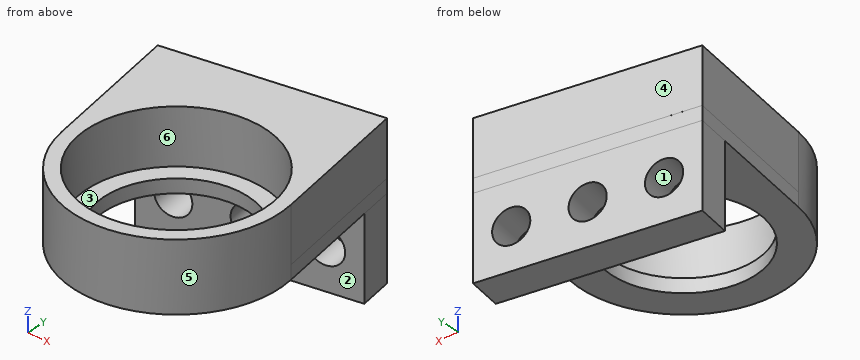
Autodesk Inventor part; units mm, degrees
ref_plane "Work Plane1" through (-17.5555, -24.5446, -8) normal (0, 0, -1) x (0, 1, 0)
ref_plane "YZ Plane" through (0, 0, 0) normal (1, 0, 0) x (0, 1, 0)
ref_plane "XZ Plane" through (0, 0, 0) normal (0, 1, 0) x (-1, 0, 0)
sketch "Sketch1" plane through (0, 0, 0) normal (0, 0, 1) x (1, 0, 0)
  circle A0 centre (0, -6.9891) radius 13
  line L0 (-8.3396, 25.9015) -> (-6.0783, 13.4045)
  line L1 (9.8647, 29.1956) -> (12.126, 16.6985)
  line L2 (-201.5028, -9.0509) -> (9.8647, 29.1956)
  line L3 (-199.2415, -21.5479) -> (-201.5028, -9.0509)
  line L4 (-199.2415, -21.5479) -> (12.126, 16.6985)
  line L5 (0, -6.9891) -> (-3.7659, 13.8229) construction
  circle A1 centre (0, -6.9891) radius 15
  line L6 (0, -6.9891) -> (-14.7603, -9.66) construction
  line L7 (-14.7603, -9.66) -> (-18.5262, 11.1521)
  line L8 (0, -6.9891) -> (14.7603, -4.3183) construction
  line L9 (14.7603, -4.3183) -> (10.9944, 16.4937)
  line L10 (10.9944, 16.4937) -> (-18.5262, 11.1521)
  point P0 (0, 0)
ref_plane "Work Plane1" through (-17.5555, -24.5446, -8) normal (0, 0, -1) x (0, 1, 0)
extrude "Extrusion1" add sketch "Sketch1" against normal up to surface (8 mm away) contours L4 L9 A1 L7 | A1
sketch "Sketch2" plane through (0, -6.9891, -8) normal (0, 0, -1) x (-0.984, -0.1781, 0)
  circle A0 centre (0, 0) radius 13
  line L0 (15, 21.15) -> (15, 0)
  line L1 (-15, 21.15) -> (15, 21.15)
  line L2 (-15, 0) -> (-15, 21.15)
  arc A1 (-15, 0) -> (15, 0) centre (0, 0) ccw
  circle A2 centre (0, 0) radius 5
  circle A3 centre (0, 0) radius 10.5
  point P0 (-1.2445, 6.8774)
extrude "Extrusion2" add sketch "Sketch2" along normal blind 2 contours A0 | L0 A1 L2 L1
ref_plane "Work Plane2" through (-83.7175, -0.6442, 79.375) normal (0.1781, -0.984, 0) x (0, 0, -1)
sketch "Sketch3" plane through (-83.7175, -0.6442, 79.375) normal (0.1781, -0.984, 0) x (0, 0, -1)
  circle A0 centre (-108.5, -103.9) radius 5
  circle A1 centre (108.5, -103.9) radius 5
  circle A2 centre (-108.5, 83.9) radius 5
  circle A3 centre (108.5, 83.9) radius 5
  arc A4 (127, 97.4) -> (122, 102.4) centre (122, 97.4) ccw
  line L0 (84.375, 102.4) -> (122, 102.4)
  arc A5 (84.375, 102.4) -> (79.375, 97.4) centre (84.375, 97.4) ccw
  line L1 (79.375, 97.4) -> (79.375, 2.8)
  line L2 (-79.375, 2.8) -> (-79.375, 97.4)
  arc A6 (-79.375, 97.4) -> (-84.375, 102.4) centre (-84.375, 97.4) ccw
  line L3 (-122, 102.4) -> (-84.375, 102.4)
  arc A7 (-122, 102.4) -> (-127, 97.4) centre (-122, 97.4) ccw
  line L4 (-127, -117.4) -> (-127, 97.4)
  arc A8 (-127, -117.4) -> (-122, -122.4) centre (-122, -117.4) ccw
  line L5 (-95, -122.4) -> (-122, -122.4)
  arc A9 (-95, -122.4) -> (-90, -117.4) centre (-95, -117.4) ccw
  line L6 (-90, -117.4) -> (-90, -47.4)
  arc A10 (-85, -42.4) -> (-90, -47.4) centre (-85, -47.4) ccw
  line L7 (-85, -42.4) -> (85, -42.4)
  arc A11 (90, -47.4) -> (85, -42.4) centre (85, -47.4) ccw
  line L8 (90, -47.4) -> (90, -117.4)
  arc A12 (90, -117.4) -> (95, -122.4) centre (95, -117.4) ccw
  line L9 (122, -122.4) -> (95, -122.4)
  arc A13 (122, -122.4) -> (127, -117.4) centre (122, -117.4) ccw
  line L10 (127, 97.4) -> (127, -117.4)
  line L11 (89.375, 66.25) -> (89.375, 96.25)
  line L12 (89.375, 96.25) -> (101.375, 96.25)
  line L13 (101.375, 96.25) -> (101.375, 66.25)
  line L14 (101.375, 66.25) -> (89.375, 66.25)
  line L15 (89.375, 66.25) -> (89.375, 96.25)
  circle A14 centre (95.375, 81.25) radius 2.5
  line L16 (95.375, 96.25) -> (95.375, 66.25)
  circle A15 centre (95.375, 71.25) radius 2.5
  circle A16 centre (95.375, 91.25) radius 2.5
  circle A17 centre (95.375, 81.25) radius 2.5
  line L17 (79.375, 66.25) -> (89.375, 66.25)
  arc A18 (77.375, 0.8) -> (79.375, 2.8) centre (77.375, 2.8) ccw
  line L18 (77.375, 0.8) -> (-77.375, 0.8)
  arc A19 (-79.375, 2.8) -> (-77.375, 0.8) centre (-77.375, 2.8) ccw
  point P0 (79.375, 82.4945)
  dimension "d5" = 12
  dimension "d6" = 5
  dimension "d9" = 10
  dimension "d12" = 10
extrude "Extrusion3" add sketch "Sketch3" along normal blind 5 contours L11 L12 L16 A16 A14 A15 L14 | L16 A15 A14 A16 L12 L13 L14
properties part number "RodBearingMount"
Work out the finished part from the listing and answer in its coordinate system (mm). Face numbers are marked on the shaded views. A direction names the side the tool comes from. Round coordinates to 2 decimals unless told otherwise and drop trailing zeros. Write each loop counter-clockwise with the first axis right and the second up, starting at its lowest first coordinate (ties: lowest second). Pieces come first, ordered by that corner, then holes. Notation, with made-up numbers: (2, -6.75) -> (55, -6.75) arc R25 ccw to (55, 18.25) -> close; hole circle Ø7 at (-4.75, 26). An arc over 180 degrees is marked (long way). Write each question's results on one line, items separated by ' | '.
Item 1: Flat-ended cylindrical pins translate along their axes: P1, Ø10, axis at x = 1, y = 2, coming from the -Z side; P2, Ø3, axis at x = 1.5, y = 14.5, coming from the +Z side; P3, Ø3, axis at x = 7, z = -9.5, coming from the +Y side; P4, Ø1, axis at x = 10, z = -5, coming from the +Y side. Find the tip coordinate at first contact, or state that the pin passes through.
Result set:
P1: z = -10 | P2: z = 0 | P3: y = 16.04 | P4: y = 16.4
Item 2: Which of the six approach directions +Z, -Z, +X, -X, +Y, -Y give full straight-line access (tool end or side, diameter ignored) to the marked faces 1, 2 and 3?
Result set:
face 1: none | face 2: -Z, +X, -Y | face 3: +Z
Item 3: A cutting plane is placed at C-C, the plane z = -18. Determine the outline of the cut face in (x, y) (1 decimal).
Result set:
outline: (-18.5, 11.2) -> (-17.6, 6.2) -> (-14.2, 6.9) -> (-15.1, 11.8) -> close; (-12.1, 12.3) -> (-11.2, 7.4) -> (-4.4, 8.6) -> (-5.2, 13.6) -> close; (-2.3, 14.1) -> (-1.4, 9.2) -> (5.5, 10.4) -> (4.6, 15.3) -> close; (7.5, 15.9) -> (8.4, 11) -> (11.9, 11.6) -> (11, 16.5) -> close
Item 4: Find the intervals of material crossed by line 1 along X through (y, z) = (-6.5, -9.25); line 2 along Y through (x, z) = (0, -9.2); line 3 along Z through (x, y) = (4.5, 7), in increasing order. Write a range as [from, to].
Result set:
line 1: [-15.33, -10.49], [10.49, 14.99] | line 2: [-21.99, -17.49], [3.51, 14.5] | line 3: [-10, 0]
Item 5: The mould has two halves that part along X. Classify the marked faces 4, 5 and 6: +X half, -X half, draft (parallel to the pull), parting line (faces both ways), or undercut.
Result set:
face 4: -X half | face 5: parting line | face 6: undercut
Item 6: A cutting plane is placed at A-A, the plane y = -14. Determine the outline of the cut face in (x, z), plus the area to 3 significant figures.
Result set:
outline: (-13.26, -10) -> (-7.82, -10) -> (-7.82, -8) -> (-10.95, -8) -> (-10.95, 0) -> (-13.26, 0) -> close; (7.82, -10) -> (13.26, -10) -> (13.26, 0) -> (10.95, 0) -> (10.95, -8) -> (7.82, -8) -> close | area: 58.8 mm^2
